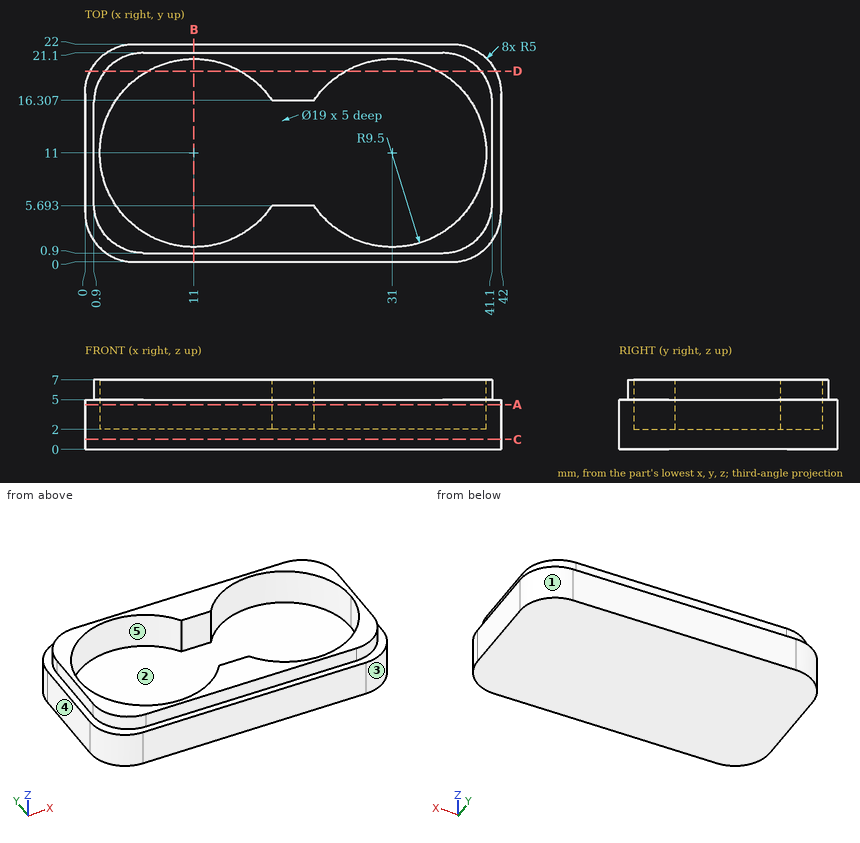
Source: three-view drawing plus pictorial views. Frame: mm from the lowest corner of the part. A direction names the side the tool comes from. Give positions to 0.01 mm unless a question says otherwise; leave off trailing zeros. Loops run counter-clockwise (first coordinate to the right, second up) from the corner with the lowest first, then second, coordinate; pieces in that order, holes last. Notation, with made-up numbers: (-23.5, -3.5) -> (19.5, -3.5) arc R13 cw to (19.5, 20.5) -> close; hole circle Ø3 at (64.25, -39.5). An arc over 180 degrees is marked (long way). Put each result on its own line as item: value. Start each with the question number.
1) Draft query along X for the marked faces 3, 4 and 5. Return one class per face: released by +X, released by -X, zero draft, split by the parting line, or undercut.
2) Contact query for flat-ended pins moving along their axis: P1, Ø3, axis at x = 16.5, y = 17.5, coming from the -Z side; P2, Ø9.5, axis at x = 13.5, y = 7, coming from the +Z side; P3, Ø1, axis at x = 25, z = 6, coming from the +Y side; P4, Ø1.6, axis at x = 19, z = 6, coming from the -Y side. Output: stop coordinate, or through.
3) Cut plane B-B (x = 11). Return loops of the section in (y, z).
4) Material intervals for probe 1 along Y at (x, z) = (11, 5.45); probe 2 along X at (y, z) = (5, 6.75) (1 decimal); probe 3 along Y at (x, z) = (11, 3.1), sorted ascending.
5) Cut plane A-A (z = 4.5). Return loops of the section in (x, y), then the cut area to 3 significant figures.
6) Cut plane C-C (z = 1). Return loops of the section in (x, y).
7) Cut plane D-D (y = 19.25). Return loops of the section in (x, z) (1 decimal), then the cut area to 3 significant figures.
8) Reachability of the marked faces 1 and 2 from +Z, -Z, +X, -X, +Y, -Y: full face, straight path, thin tool, end or side. Return the list, or none.
Results are:
1. face 3: released by +X
1. face 4: released by -X
1. face 5: undercut
2. P1: stops at z = 0
2. P2: stops at z = 2
2. P3: stops at y = 21.1
2. P4: stops at y = 0.9
3. outline: (0, 0) -> (22, 0) -> (22, 5) -> (21.1, 5) -> (21.1, 7) -> (20.5, 7) -> (20.5, 2) -> (1.5, 2) -> (1.5, 7) -> (0.9, 7) -> (0.9, 5) -> (0, 5) -> close
4. probe 1: y = 0.9 to 1.5, 20.5 to 21.1
4. probe 2: x = 1 to 3.6, 18.4 to 23.6, 38.4 to 41
4. probe 3: y = 0 to 1.5, 20.5 to 22
5. outline: (0, 5) arc R5 ccw to (5, 0) -> (37, 0) arc R5 ccw to (42, 5) -> (42, 17) arc R5 ccw to (37, 22) -> (5, 22) arc R5 ccw to (0, 17) -> close; hole (18.88, 5.69) -> (23.12, 5.69) arc R9.5 ccw to (40.5, 11) arc R9.5 ccw to (23.12, 16.31) -> (18.88, 16.31) arc R9.5 ccw (long way) to start
5. area: 314 mm2
6. outline: (0, 5) arc R5 ccw to (5, 0) -> (37, 0) arc R5 ccw to (42, 5) -> (42, 17) arc R5 ccw to (37, 22) -> (5, 22) arc R5 ccw to (0, 17) -> close
7. outline: (0.5, 0) -> (41.5, 0) -> (41.5, 5) -> (40, 5) -> (40, 7) -> (35.7, 7) -> (35.7, 2) -> (26.3, 2) -> (26.3, 7) -> (15.7, 7) -> (15.7, 2) -> (6.3, 2) -> (6.3, 7) -> (2, 7) -> (2, 5) -> (0.5, 5) -> close
7. area: 186 mm2
8. face 1: +Z, -Z, +X, +Y
8. face 2: +Z
